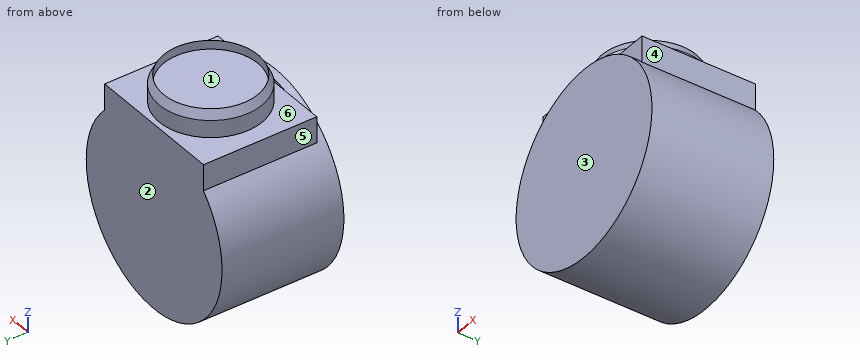
from build123d import *

# Parameters (mm, degrees)
SKETCH1_R           = 55
BOSS_EXTRUDE1_DEPTH = 66
BOSS_EXTRUDE3_DEPTH = 63
SKETCH5_R           = 56.242985336
SKETCH5_R_2         = 30
CUT_EXTRUDE2_DEPTH  = 10
BOSS_EXTRUDE4_START = 5
SKETCH6_R           = 55
BOSS_EXTRUDE4_DEPTH = 5


with BuildPart() as part:
    # Sketch1 → Boss-Extrude1 (new body)
    with BuildSketch(Plane(origin=(0, 0, 0), x_dir=(1, 0, 0), z_dir=(0, 1, 0))):
        with Locations(Location((0, 0, 0), (0, 0, 270))):
            Circle(SKETCH1_R)
    extrude(amount=BOSS_EXTRUDE1_DEPTH)

    # Sketch2 → Boss-Extrude3 (add)
    with BuildSketch(Plane.XY):
        Polygon((-40, 66), (-40, 0), (0, 0), (40, 0), (40, 66), align=None)
    extrude(amount=BOSS_EXTRUDE3_DEPTH)

    # Sketch4 → Revolve1 (revolve)
    with BuildSketch(Plane(origin=(0, 0, 0), x_dir=(0, 0, -1), z_dir=(1, 0, 0)), mode=Mode.PRIVATE) as revolve1_sk:
        Polygon((-63, 5.5), (-68.077040766, 5.5), (-63, 3), align=None)
    revolve(revolve1_sk.sketch.rotate(Axis((0, 33, 63), (0, 0, 1)), 270), axis=Axis((0, 33, 63), (0, 0, 1)))

    # Sketch5 → Cut-Extrude2 (cut)
    with BuildSketch(Plane.XY.offset(63)):
        with Locations((0, 33)):
            Circle(SKETCH5_R)
        with Locations((0, 33)):
            Circle(SKETCH5_R_2, mode=Mode.SUBTRACT)
    extrude(amount=-CUT_EXTRUDE2_DEPTH, mode=Mode.SUBTRACT)

    # Sketch6 → Boss-Extrude4 (add)
    with BuildSketch(Plane(origin=(0, 0, 0), x_dir=(-1, 0, 0), z_dir=(0, -1, 0)).offset(BOSS_EXTRUDE4_START)):
        with Locations(Location((0, 0, 0), (0, 0, 90))):
            Circle(SKETCH6_R)
    extrude(amount=-BOSS_EXTRUDE4_DEPTH)


solid = part.part
CAD build for the part. Positions are in the model's coordinates, mm. Face numbers are marked on the shaded views. A direction names the side the tool comes from. Give positions to 0.01 mm unless a question says otherwise; leave off trailing zeros. Write each loop counter-clockwise with the first axis right and the second up, starting at its lowest first coordinate (ties: lowest second). Pieces come first, ordered by that corner, then holes. Notation, with made-up numbers: M 44,55.25 L 62,55.25 A24 ccw 62,77.25 Z; hole C 38.25,-12 d5. An arc over 180 degrees is marked long. Put each result on its own line as item: value. Start each with the question number.
(1) Band-saw the part on A-A, the plane y = 33. Write the cut outline in (x, z).
(2) Mould opens along Y. For the marked faces 1, 2, 3 and 4 say: +Y half, -Y half, draft (parallel to the pull), parting line (faces both ways), or undercut.
(3) Band-saw the part on B-B, the plane z = 50.5. Write the cut outline in (x, y).
(4) Band-saw the part on C-C, the plane x = 0. Write the cut outline in (y, z), and give its area (3 significant figures).
(5) Probe L1, parallel to X at y = 16.5, z = 42; L2, parallel to Y at x = 0, z = 66.5; L3, parallel to Y at x = 0, z = 65. List the from-to ranges inside material, lowest first.
(6) Flat gauge pins, fed straight in: pin 1 Ø7.5 at (y, z) = (35, 48) entering from -X; pin 2 Ø4 at (y, z) = (3, 23) entering from -X; pin 3 Ø12 at (y, z) = (6, 8) entering from -X. Where does each tip first touch, or does it go through?
(7) Band-saw the part on D-D, the plane z = 35. Write the cut outline in (x, y), and give its area (3 significant figures).
(8) Which spindle directions (+Z, -Z, +X, -X, +Y, -Y) get a long thin tool onto all of the face, cutting with end or side? Do the marked faces 5 and 6. Say none if no direction does.
Response values:
1. outline: M -40,37.75 A55 ccw long 40,37.75 L 40,53 L 30,53 L 30,63 L 27.5,68.08 L 27.5,63 L -27.5,63 L -27.5,68.08 L -30,63 L -30,53 L -40,53 Z
2. face 1: undercut
2. face 2: +Y half
2. face 3: -Y half
2. face 4: draft
3. outline: M -40,0 L -21.79,0 L -21.79,-5 L 21.79,-5 L 21.79,0 L 40,0 L 40,66 L -40,66 Z
4. outline: M -5,-55 L 66,-55 L 66,53 L 63,53 L 63,63 L 60.5,68.08 L 60.5,63 L 5.5,63 L 5.5,68.08 L 3,63 L 3,53 L 0,53 L 0,55 L -5,55 Z
4. area: 8,290 mm2
5. L1: x = -40 to 40
5. L2: y = 4.72 to 5.5, 60.5 to 61.28
5. L3: y = 3.98 to 5.5, 60.5 to 62.02
6. pin 1: stops at x = -40
6. pin 2: stops at x = -50.83
6. pin 3: stops at x = -54.96
7. outline: M -42.43,-5 L 42.43,-5 L 42.43,66 L -42.43,66 Z
7. area: 6,020 mm2
8. face 5: +Z, -X, +Y, -Y
8. face 6: +Z
